The listing builds one solid part. Answer for the finished solid, in the listing's coordinates (mm). Face numbers are marked on the shaded views. A direction names the side the tool comes from. Coordinates: 2 decimals unless noted, no trailing zeros. Write each loop counter-clockwise with the first axis right and the second up, starting at its lowest first coordinate (ties: lowest second). Pieces come first, ordered by that corner, then holes. Notation, with made-up numbers: M 3,15 L 33,15 A20 ccw 33,24 Z; hole C 12,0 d10. An arc over 180 degrees is marked long. Write item = value, one per line. Start each with the question number.
```python
from build123d import *

# Parameters (mm, degrees)
SKETCH1_R               = 2
EXTRUDE1_DEPTH          = 40
CUT_EXTRUDE1_DEPTH      = 5
CUT_EXTRUDE1_DEPTH_BACK = 6
HOLE1_AT_2_COUNT        = 2
HOLE1_AT_2_PITCH        = 25


with BuildPart() as part:
    # Sketch1 → Extrude1 (new body)
    with BuildSketch(Plane.XY):
        with BuildLine():
            Line((-31.475233645, -9.996703011), (-15.475233645, -9.996703011))
            Line((-15.475233645, -9.996703011), (-15.475233645, -9.496703011))
            Line((-15.475233645, -9.496703011), (-11.475233645, -9.496703011))
            ThreePointArc((-11.475233645, -9.496703011), (-7.939699739, -8.032236917), (-6.475233645, -4.496703011))
            Line((-6.475233645, -4.496703011), (-6.475233645, -3.996703011))
            Line((-6.475233645, -3.996703011), (-9.475233645, -0.996703011))
            Line((-9.475233645, -0.996703011), (-13.475233645, -0.996703011))
            Line((-13.475233645, -0.996703011), (-16.475233645, -3.996703011))
            Line((-16.475233645, -3.996703011), (-16.475233645, -4.996703011))
            Line((-16.475233645, -4.996703011), (-29.075233645, -4.996703011))
            Line((-29.075233645, -4.996703011), (-31.475233645, -7.396703011))
            Line((-31.475233645, -7.396703011), (-31.475233645, -9.996703011))
        make_face()
        with Locations((-11.475233645, -3.996703011)):
            Circle(SKETCH1_R, mode=Mode.SUBTRACT)
    extrude(amount=EXTRUDE1_DEPTH)

    # Sketch2 → Cut-Extrude1 (cut, two sides)
    with BuildSketch(Plane(origin=(0, -4.996703011, 0), x_dir=(1, 0, 0), z_dir=(0, 1, 0))) as cut_extrude1_sk:
        Polygon((-9.475233645, -20), (-16.975233645, -20), (-16.975233645, -28.700140492), (-16.975233645, -30), (-3.073130332, -30), (-3.073130332, -20), align=None)
        Polygon((-9.475233645, -10), (-16.975233645, -10), (-16.975233645, 0), (-9.475233645, 0), (-4.909711278, 0), (-4.909711278, -10), align=None)
    extrude(amount=CUT_EXTRUDE1_DEPTH, mode=Mode.SUBTRACT)
    extrude(cut_extrude1_sk.sketch, amount=-CUT_EXTRUDE1_DEPTH_BACK, mode=Mode.SUBTRACT)

    # Sketch4 → Hole1 (revolve, cut)
    with BuildSketch(Plane(origin=(-23.975233645, -4.996703011, 7.5), x_dir=(0, 0, 1), z_dir=(1, 0, 0))):
        Polygon((0, 0), (0, 5), (2.6, 5), (2.6, 2.5), (5.1, 0), align=None)
    hole1 = revolve(axis=Axis((-23.975233645, 1.353296989, 7.5), (0, -1, 0)), mode=Mode.SUBTRACT)

    # Hole1 at 2: Hole1 ×2
    with Locations(*[(0, 0, i * HOLE1_AT_2_PITCH) for i in range(1, HOLE1_AT_2_COUNT)]):
        add(hole1, mode=Mode.SUBTRACT)


solid = part.part
```
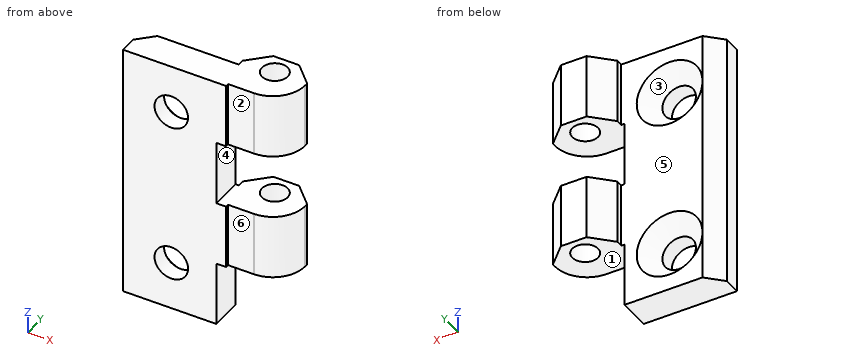
1. The part is cut by section D-D, the plane y = -8.5. Write down the section's boundary in (x, z).
2. Straight lines are drawn through the part: L1, parallel to Z at x = -10.5, y = -7.75; L2, parallel to X at y = -8.9, z = 7.5; L3, parallel to Y at x = -13, z = 32. For each, find the intervals that lie inside material, in ascending order. Write a range as [from, to].
3. For a pull along Z with two mould halves and no side action, classify the marked faces 1, 2 and 3 as pulls with the +Z half, pulls with the -Z half, needs draft (parallel to the pull), parting line crosses it, or undercut.
4. For the marked faces 4, 5 and 6, determine the directions among +Z, -Z, +X, -X, +Y, -Y from which every point of the face is accessible in a straight line to the end or side of a thin tool.
5. The part is cut by section A-A, the plane z = 16.5. Write down the section's boundary in (x, y).
6. The part is cut by section B-B, the plane y = -3.25. Write down the section's boundary in (x, z).
7. Each of these flat-tipped pins is pushed along its axis until it touches: pin 1 (0.5 mm diameter, centred on y = -4.5, z = 37, fed in from -X); pin 2 (1 mm diameter, centred on x = -12.5, y = -5.5, fed in from -Z); pin 3 (10 mm diameter, centred on x = -21, z = 13, fed in from +Y); pin 4 (4.5 mm diameter, centred on x = -11.48, y = -4, fed in from +Z). Where does it stop, or does it pass through?
8. The part is cut by section C-C, the plane z = 27. Write down the section's boundary in (x, y), and give its area (3 significant figures).
Solution:
q1.outline = M -31.48,0 L -16.98,0 L -16.98,10 L -8.48,10 L -8.48,20 L -16.98,20 L -16.98,30 L -8.48,30 L -8.48,40 L -31.48,40 Z; hole C -23.98,7.5 d5.2; hole C -23.98,32.5 d5.2
q2.L1 = [10, 20], [30, 40]
q2.L2 = [-31.48, -26.58], [-21.38, -16.98]
q2.L3 = [-9.5, -5.29], [-2.7, -1]
q3.face_1 = pulls with the -Z half
q3.face_2 = needs draft
q3.face_3 = undercut
q4.face_4 = +X, +Y, -Y
q4.face_5 = +Z, -Z, -X, +Y
q4.face_6 = +Z, -Z, +X, -Y
q5.outline = M -31.48,-10 L -15.48,-10 L -15.48,-9.5 L -11.48,-9.5 A5 ccw -6.48,-4.5 L -6.48,-4 L -9.48,-1 L -13.48,-1 L -16.48,-4 L -16.48,-5 L -29.08,-5 L -31.48,-7.4 Z; hole C -11.48,-4 d4
q6.outline = M -15.73,10 L -13.33,10 L -13.33,20 L -15.73,20 Z; M -15.73,30 L -13.33,30 L -13.33,40 L -15.73,40 Z; M -9.62,10 L -7.22,10 L -7.22,20 L -9.62,20 Z; M -9.62,30 L -7.22,30 L -7.22,40 L -9.62,40 Z
q7.pin_1 = -16.48
q7.pin_2 = 10
q7.pin_3 = -3.52
q7.pin_4 = 40
q8.outline = M -31.48,-10 L -16.98,-10 L -16.98,-5 L -29.08,-5 L -31.48,-7.4 Z
q8.area = 69.6 mm^2
